For this review, take the finished solid that the model builds, in its own axes (mm). Face numbers are marked on the shaded views. A direction names the side the tool comes from. Give positions to 0.01 mm unless a question says otherwise; leave off trailing zeros. Order: outer loops, then holes, each group sorted by start corner. A loop starts at its lowest first (then second) coordinate and runs counter-clockwise, first axis right, second up. Notation, with made-up numbers: M 80,39 L 113,39 A24 cw 113,74 Z; hole C 12.5,69 d6. An arc over 180 degrees is marked long. Answer as CSV lines item,"result". Start each with the question number.
1. Clearance check with flat-ended pins moving along their axes: P1, Ø3, axis at x = 41.5, z = 2.5, coming from the -Y side; P2, Ø2.5, axis at y = -1.5, z = -15, coming from the -X side (3 decimals); P3, Ø1.5, axis at y = -2, z = 15.5, coming from the +X side (3 decimals). State where each tip first meets the part, or that it passes through.
2. Machinability: for the marked faces 1 and 2, which of the approach directions +Z, -Z, +X, -X, +Y, -Y give a long, thin tool a straight path to every point of the face, cutting with its end or side? Answer none if there is none.
3. We need section C-C, the plane x = -7.5. Give the boundary of the cut face in (y, z) (3 decimals), and give its area (3 significant figures).
4. We need section B-B, the plane y = -3.75. Give the boundary of the cut face in (x, z) (3 decimals).
5. For line 1 along Z through (x, y) = (-52.5, -3.5) (3 decimals); line 2 along Y through (x, z) = (-49.5, 16.5); line 3 along X through (y, z) = (-3.25, 12) (3 decimals), list the stretches that pass through material, from the lowest coordinate up.
6. We need section A-A, the plane z = -7.5. Give the boundary of the cut face in (x, y) (3 decimals).
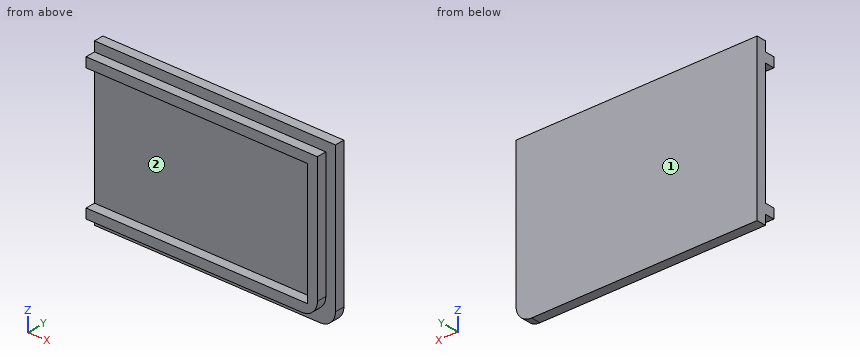
from build123d import *

# Parameters (mm, degrees)
SALIENTE_EXTRUIR1_DEPTH = 5
SALIENTE_EXTRUIR2_DEPTH = 5


with BuildPart() as part:
    # Croquis1 → Saliente-Extruir1 (new body)
    with BuildSketch(Plane(origin=(0, 0, 0), x_dir=(1, 0, 0), z_dir=(0, 1, 0))):
        with BuildLine():
            Line((-62.245, -41.575), (62.245, -41.575))
            Line((62.245, -41.575), (62.245, 33.575))
            ThreePointArc((62.245, 33.575), (59.901854249, 39.231854249), (54.245, 41.575))
            Line((54.245, 41.575), (-62.245, 41.575))
            Line((-62.245, 41.575), (-62.245, -41.575))
        make_face()
    extrude(amount=SALIENTE_EXTRUIR1_DEPTH)

    # Croquis2 → Saliente-Extruir2 (add)
    with BuildSketch(Plane(origin=(0, 0, 0), x_dir=(1, 0, 0), z_dir=(0, 1, 0))):
        with BuildLine():
            Line((52.245, -31.575), (52.245, 31.575))
            Line((52.245, 31.575), (21.4, 31.575))
            Line((21.4, 31.575), (-62.245, 31.575))
            Line((-62.245, 31.575), (-62.245, 36.575))
            Line((-62.245, 36.575), (49.245, 36.575))
            ThreePointArc((49.245, 36.575), (54.901854249, 34.231854249), (57.245, 28.575))
            Line((57.245, 28.575), (57.245, -36.575))
            Line((57.245, -36.575), (-62.245, -36.575))
            Line((-62.245, -36.575), (-62.245, -31.575))
            Line((-62.245, -31.575), (52.245, -31.575))
        make_face()
    extrude(amount=-SALIENTE_EXTRUIR2_DEPTH)


solid = part.part
Result set:
1,P1,"y = 0"
1,P2,"x = 52.245"
1,P3,"x = 57.245"
2,face 1,"+Z, -Z, +X, -X, +Y"
2,face 2,"-X, -Y"
3,outline,"M -5,-36.575 L 0,-36.575 L 0,-41.575 L 5,-41.575 L 5,41.575 L 0,41.575 L 0,36.575 L -5,36.575 L -5,31.575 L 0,31.575 L 0,-31.575 L -5,-31.575 Z"
3,area,"466 mm2"
4,outline,"M -62.245,-36.575 L 49.245,-36.575 A8 ccw 57.245,-28.575 L 57.245,36.575 L -62.245,36.575 L -62.245,31.575 L 52.245,31.575 L 52.245,-31.575 L -62.245,-31.575 Z"
5,line 1,"-36.575 to -31.575, 31.575 to 36.575"
5,line 2,"0 to 5"
5,line 3,"52.245 to 57.245"
6,outline,"M -62.245,0 L 52.245,0 L 52.245,-5 L 57.245,-5 L 57.245,0 L 62.245,0 L 62.245,5 L -62.245,5 Z"
